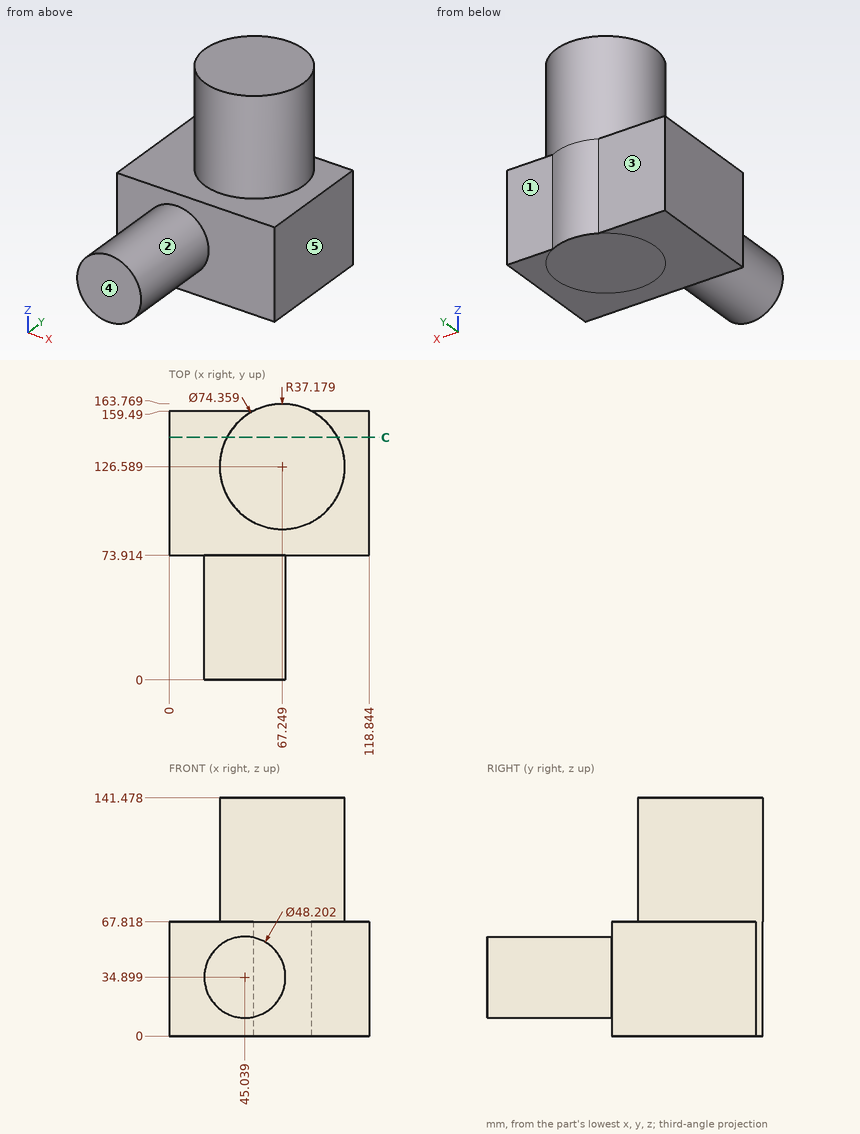
Geometry check sheet. Reference: drawing and pictorial views, mm from the part's lowest x, y, z. A direction names the side the tool comes from. Give positions to 0.01 mm unless a question says otherwise; leave off trailing zeros. Write each loop counter-clockwise with the first axis right and the second up, starting at its lowest first coordinate (ties: lowest second). Pieces come first, ordered by that corner, then holes. Notation, with made-up numbers: (-13, -0.75) -> (0, -0.75) arc R5 cw to (0, 3.25) -> close; hole circle Ø1 at (-2, -19.5). An arc over 180 degrees is marked (long way). One line per item, written item: value. Start each with the question number.
Item 1: Section check C-C on y = 144. Record the cut outline in (x, z) (1 decimal), then the cut area to 3 significant figures.
Item 2: Tool access check on the marked faces 1, 2, 3, 4 and 5. Record the directions out of +Z, -Z, +X, -X, +Y, -Y that give a thin tool (end or side, any length) a straight path to the whole face; none if there is none.
Item 3: Material ranges on probe 1 along Y at (x, z) = (112, 17) (1 decimal); probe 2 along Z at (x, y) = (106, 122); probe 3 along Y at (x, z) = (68.5, 123), recorded low to high. Write a range as from..to.
Item 4: Gauge pin test, flat ends, axial feed: pin 1 (8 mm diameter, centred on x = 64, y = 72.5, fed in from +Z); pin 2 (2 mm diameter, centred on x = 40, y = 22, fed in from +Z); pin 3 (5 mm diameter, centred on x = 74, z = 40.5, fed in from +Y) (1 decimal). Record the tip position at first contact, or that the pin passes through.
Results list:
1. outline: (0, 0) -> (118.8, 0) -> (118.8, 67.8) -> (100.1, 67.8) -> (100.1, 141.5) -> (34.4, 141.5) -> (34.4, 67.8) -> (0, 67.8) -> close
1. area: 12,900 mm²
2. face 1: +Z, -Z, +X, +Y
2. face 2: -Y
2. face 3: +Z, -Z, -X, +Y
2. face 4: +Z, -Z, +X, -X, -Y
2. face 5: +Z, -Z, +X, +Y, -Y
3. probe 1: 73.9..159.5
3. probe 2: 0..67.82
3. probe 3: 89.43..163.75
4. pin 1: z = 67.82
4. pin 2: z = 58.66
4. pin 3: y = 163.5
